Source: CAD feature listing. Evaluate the final solid. Frame: model axes, mm. A direction names the side the tool comes from. Round coordinates to 2 decimals unless told otherwise and drop trailing zeros. Order: outer loops, then holes, each group sorted by start corner. A loop starts at its lowest first (then second) coordinate and runs counter-clockwise, first axis right, second up. Notation, with made-up numbers: M 76.25,-29 L 118.25,-29 A12 ccw 118.25,-8 Z; hole C -18.75,88 d2. An arc over 180 degrees is marked long. Use one line per item in the form item = value. Start each with the question number.
Q1. Material intervals for probe 1 along Y at (x, z) = (14, 21.5); probe 2 along Z at (x, y) = (2.5, 107.5); probe 3 along X at (y, z) = (46, 0), sorted ascending.
Q2. Contact query for flat-ended pins moving along their axis: pin 1 (1.8 mm diameter, centred on y = 100.5, z = 21, fed in from +X); pin 2 (5 mm diameter, centred on x = -5, z = 21, fed in from -Y); pin 3 (3 mm diameter, centred on x = 0.5, z = 21.5, fed in from -Y). Output: stop coordinate, or through.
Q3. Section C-C (z = -7). Return the cut outline in (x, y), plus the area to 3 significant figures.
Q4. Reachability of faces 4 (the flat face through (0, 5, 10.5)), 5 (the flat face through (-17, 82, 20)), 6 (the flat face through (20, 70, 13)), 7 (the flat face through (13, 70, -0.5)) from +Z, -Z, +X, -X, +Y, -Y: full face, straight path, thin tool, end or side. Return the list, or none.
Q5. Section A-A (x = 0). Return the cut outline in (y, z).
Q6. Section D-D (x = 6). Return the cut outline in (y, z), plus the area to 3 significant figures.
Q7. Section B-B (y = 20.5). Return the cut outline in (x, z).
Q8. Pull-direction query (Z, two-part tool) for faces 1 (the cylindrical face through (18.57, 72.5, 1)), 2 (the flat face through (2, 133, 20)), 3 (the cylindrical face through (0.28, 16.294, 13.066)); classes: pulls with the +Z half, pulls with the -Z half, needs draft (parallel to the pull), parting line crosses it, or undercut.
from build123d import *

# Parameters (mm, degrees)
SKETCH1_R           = 9.25
BOSS_EXTRUDE1_DEPTH = 143
FILLET2_R           = 5
SKETCH2_W           = 6
SKETCH2_H           = 103
CUT_EXTRUDE1_DEPTH  = 37
FILLET3_R           = 5
CUT_EXTRUDE2_DEPTH  = 53


with BuildPart() as part:
    # Sketch1 → Boss-Extrude1 (new body)
    with BuildSketch(Plane(origin=(0, 0, 0), x_dir=(1, 0, 0), z_dir=(0, 1, 0))):
        with BuildLine():
            Line((0, -26), (-20, -26))
            Line((-20, -26), (-20, -4.5))
            Line((-20, -4.5), (-20, -2.5))
            Line((-20, -2.5), (-20, 0.5))
            Line((-20, 0.5), (-17, 0.5))
            Line((-17, 0.5), (-11.238883396, 0.5))
            ThreePointArc((-11.238883396, 0.5), (0, 11.25), (11.238883396, 0.5))
            Line((11.238883396, 0.5), (17, 0.5))
            Line((17, 0.5), (20, 0.5))
            Line((20, 0.5), (20, -2.5))
            Line((20, -2.5), (20, -4.5))
            Line((20, -4.5), (20, -26))
            Line((20, -26), (0, -26))
        make_face()
        Circle(SKETCH1_R, mode=Mode.SUBTRACT)
    extrude(amount=BOSS_EXTRUDE1_DEPTH)

    # Fillet2
    fillet2_edges = [part.edges().sort_by_distance(p)[0] for p in [
        (-20, 71.5, -0.5),
        (20, 71.5, -0.5),
    ]]
    fillet(fillet2_edges, radius=FILLET2_R)

    # Sketch2 → Cut-Extrude1 (cut)
    with BuildSketch(Plane(origin=(20, 0, 0), x_dir=(0, 0, -1), z_dir=(1, 0, 0))):
        with Locations((-20, 81.5)):
            Rectangle(SKETCH2_W, SKETCH2_H)
    extrude(amount=-CUT_EXTRUDE1_DEPTH, mode=Mode.SUBTRACT)

    # Fillet3
    fillet3_edges = [part.edges().sort_by_distance(p)[0] for p in [
        (0, 0, 26),
        (0, 143, 26),
    ]]
    fillet(fillet3_edges, radius=FILLET3_R)

    # Sketch3 → Cut-Extrude2 (cut)
    with BuildSketch(Plane(origin=(20, 0, 0), x_dir=(0, 0, -1), z_dir=(1, 0, 0))):
        with BuildLine():
            Line((-10.5, 0), (-10.5, 10))
            ThreePointArc((-10.5, 10), (-13.136038969, 16.363961031), (-19.5, 19))
            Line((-19.5, 19), (-26, 19))
            Line((-26, 19), (-26, 5))
            ThreePointArc((-26, 5), (-24.535533906, 1.464466094), (-21, 0))
            Line((-21, 0), (-10.5, 0))
        make_face()
    extrude(amount=-CUT_EXTRUDE2_DEPTH, mode=Mode.SUBTRACT)


solid = part.part
Results list:
q1.probe_1 = 19 to 30, 133 to 142.97
q1.probe_2 = -10.97 to -8.91, 8.91 to 17, 23 to 26
q1.probe_3 = -17.18 to -9.25, 9.25 to 17.18
q2.pin_1 = -17
q2.pin_2 = 18.94
q2.pin_3 = 19
q3.outline = M -8.81,0 L -6.05,0 L -6.05,143 L -8.81,143 Z; M 6.05,0 L 8.81,0 L 8.81,143 L 6.05,143 Z
q3.area = 789 mm2
q4.face_4 = +Z, +X, -X, -Y
q4.face_5 = +X
q4.face_6 = +Z, -Z, +X, +Y, -Y
q4.face_7 = -Z, +X, +Y, -Y
q5.outline = M 0,-11.25 L 143,-11.25 L 143,-9.25 L 0,-9.25 Z; M 0,9.25 L 143,9.25 L 143,21 A5 ccw 138,26 L 19,26 L 19,19.5 A9 cw 10,10.5 L 0,10.5 Z; hole M 30,17 L 133,17 L 133,23 L 30,23 Z
q6.outline = M 0,-9.52 L 143,-9.52 L 143,-7.04 L 0,-7.04 Z; M 0,7.04 L 143,7.04 L 143,21 A5 ccw 138,26 L 19,26 L 19,19.5 A9 cw 10,10.5 L 0,10.5 Z; hole M 30,17 L 133,17 L 133,23 L 30,23 Z
q6.area = 2,160 mm2
q7.outline = M -20,4.5 A5 ccw -15,-0.5 L -11.24,-0.5 A11.25 ccw 11.24,-0.5 L 15,-0.5 A5 ccw 20,4.5 L 20,26 L -20,26 Z; hole C 0,0 d18.5
q8.face_1 = pulls with the -Z half
q8.face_2 = undercut
q8.face_3 = pulls with the +Z half
